```python
from build123d import *

# Parameters (mm, degrees)
SKETCH2_R          = 6
CONE_DEPTH         = 8
CONE_TAPER         = 36
SKETCH5_R          = 2.825
CUT_EXTRUDE3_DEPTH = 13
SKETCH4_W          = 5.5
SKETCH4_H          = 5.3
CUT_EXTRUDE2_DEPTH = 8
SKETCH6_R          = 2.55
CUT_EXTRUDE4_DEPTH = 10


with BuildPart() as part:
    # Sketch1 → Revolve1 (revolve)
    with BuildSketch(Plane(origin=(0, 0, 0), x_dir=(1, 0, 0), z_dir=(0, 1, 0))):
        with BuildLine():
            Line((0, -12), (0, 12))
            ThreePointArc((0, 12), (12, 0), (0, -12))
        make_face()
    revolve(axis=Axis((0, 0, 12), (0, 0, -1)))

    # Sketch2 → Cone (cut)
    with BuildSketch(Plane.XY.offset(12)):
        Circle(SKETCH2_R)
    extrude(amount=-CONE_DEPTH, taper=CONE_TAPER, mode=Mode.SUBTRACT)

    # Sketch5 → Cut-Extrude3 (cut)
    with BuildSketch(Plane(origin=(0, 0, -12), x_dir=(-1, 0, 0), z_dir=(0, 0, -1))):
        Circle(SKETCH5_R)
    extrude(amount=-CUT_EXTRUDE3_DEPTH, mode=Mode.SUBTRACT)

    # Sketch4 → Cut-Extrude2 (cut)
    with BuildSketch(Plane(origin=(0, -12, 0), x_dir=(-1, 0, 0), z_dir=(0, -1, 0))):
        Rectangle(SKETCH4_W, SKETCH4_H)
    extrude(amount=-CUT_EXTRUDE2_DEPTH, mode=Mode.SUBTRACT)

    # Sketch6 → Cut-Extrude4 (cut)
    with BuildSketch(Plane(origin=(0, 0, 1), x_dir=(-1, 0, 0), z_dir=(0, 0, -1))):
        Circle(SKETCH6_R)
    extrude(amount=-CUT_EXTRUDE4_DEPTH, mode=Mode.SUBTRACT)


solid = part.part
```
Verification items for the finished model (mm, model axes). A direction names the side the tool comes from. Coordinates: 2 decimals unless noted, no trailing zeros. Loops run counter-clockwise (first coordinate to the right, second up) from the corner with the lowest first, then second, coordinate; pieces in that order, holes last. Notation, with made-up numbers: (76.5, 11.5) - (129.5, 11.5) arc R30 cw to (129.5, 36.5) - close; hole circle Ø6 at (60, 67.5). An arc over 180 degrees is marked (long way). Return JSON: item names as keys, results as strings.
1. Section check B-B, the plane y = -7. Record the boundary of the cut face in (x, z).
Established:
{"outline": "circle Ø19.49 at (0, 0); hole (-2.75, -2.65) - (2.75, -2.65) - (2.75, 2.65) - (-2.75, 2.65) - close"}
2. Mould release check, pull along Y, two halves, no side actions. Record for faces 4 (the conical face through (-0.58, -2.613, 7.426)), 5 (the flat face through (0, -4, 0)), 6 (the flat face through (0, -8, 2.65)): +Y half, -Y half, draft (parallel to the pull), parting line (faces both ways), or undercut.
Established:
{"face 4": "undercut", "face 5": "-Y half", "face 6": "draft"}
3. Go/stop test with flat-tipped pins: pin 1 (8 mm diameter, centred on x = 0, y = 0, fed in from +Z); pin 2 (1.7 mm diameter, centred on x = 0.5, y = -7, fed in from +Z); pin 3 (2.5 mm diameter, centred on x = 1, z = 0, fed in from -Y); pin 4 (4.5 mm diameter, centred on x = 0, y = 0, fed in from -Z). Record where each tip stops, or that it passes through.
Established:
{"pin 1": "stops at z = 9.25", "pin 2": "stops at z = 10.29", "pin 3": "stops at y = -4", "pin 4": "passes through"}
4. Section check D-D, the plane x = 9. Record the boundary of the cut face in (y, z), then the cut area to 3 significant figures.
Established:
{"outline": "circle Ø15.87 at (0, 0)", "area": "198 mm2"}
5. Tool access check on faces 1 (the flat face through (-2.75, -8, 0)), 2 (the cylindrical face through (-1.18, -2.26, 4.08)), 3 (the cylindrical face through (-2.695, 0.849, -5.42)). Record the directions out of +Z, -Z, +X, -X, +Y, -Y that give a thin tool (end or side, any length) a straight path to the whole face; none if there is none.
Established:
{"face 1": "-Y", "face 2": "+Z, -Z", "face 3": "-Z"}
6. Thickness scan on L1, parallel to Z at x = -1, y = -10.25; L2, parallel to X at y = 0, z = 4.75; L3, parallel to Y at x = 0, z = -3.25 (3 decimals). Record the ranges inside material, lowest first.
Established:
{"L1": "z = -6.16 to -2.65, 2.65 to 6.16", "L2": "x = -11.02 to -2.55, 2.55 to 11.02", "L3": "y = -11.552 to -2.825, 2.825 to 11.552"}
7. Section check A-A, the plane x = 0. Record the boundary of the cut face in (y, z) (3 decimals), then the cut area to 3 significant figures.
Established:
{"outline": "(-11.704, -2.65) arc R12 ccw to (-2.825, -11.663) - (-2.825, 1) - (-2.55, 1) - (-2.55, 7.251) - (-5.155, 10.836) arc R12 ccw to (-11.704, 2.65) - (-4, 2.65) - (-4, -2.65) - close; (2.55, 1) - (2.825, 1) - (2.825, -11.663) arc R12 ccw to (5.155, 10.836) - (2.55, 7.251) - close", "area": "270 mm2"}
8. Section check C-C, the plane z = -3.25. Record the boundary of the cut face in (x, y) (3 decimals), then the cut area to 3 significant figures.
Established:
{"outline": "circle Ø23.103 at (0, 0); hole circle Ø5.65 at (0, 0)", "area": "394 mm2"}
